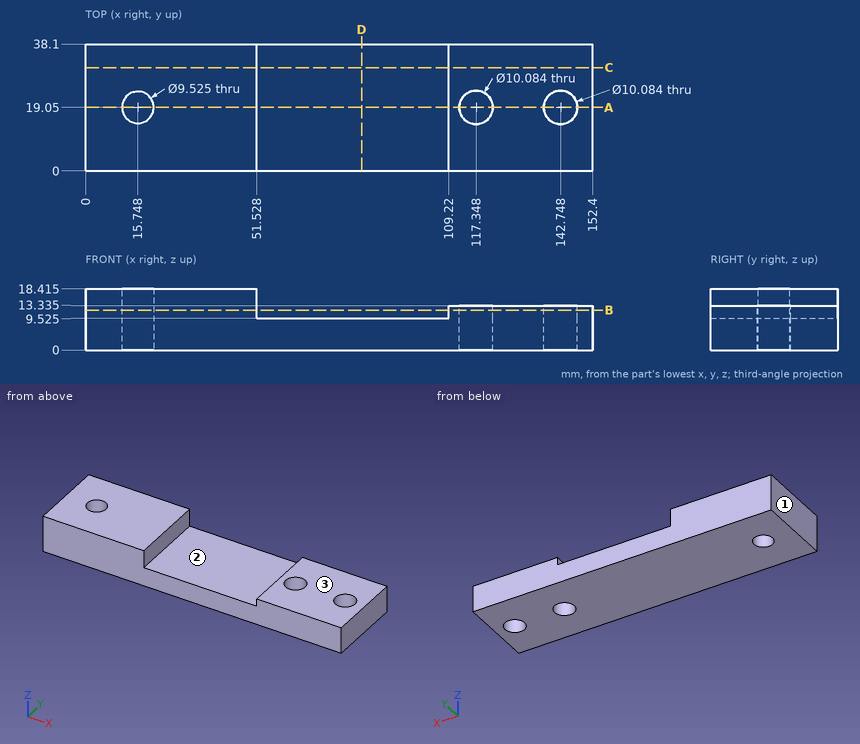
For this review, use the dimensioned drawing (mm, ordinates from the lowest corner) and the shaded views. A direction names the side the tool comes from. Round coordinates to 2 decimals unless told otherwise and drop trailing zeros. Write each loop counter-clockwise with the first axis right and the second up, starting at its lowest first coordinate (ties: lowest second). Pieces come first, ordered by that corner, then holes. Notation, with made-up numbers: (-1.75, -30.75) - (57.25, -30.75) arc R7 ccw to (57.25, -23.75) - close; hole circle Ø10 at (52, 23). An arc over 180 degrees is marked (long way). Use a Markdown table: item, result.
Q1. Machinability: for the marked faces 1, 2 and 3, which of the approach directions +Z, -Z, +X, -X, +Y, -Y give a long, thin tool a straight path to every point of the face, cutting with its end or side? Answer none if there is none.
Derived:
| item | result |
|---|---|
| face 1 | +Z, -Z, -X, +Y, -Y |
| face 2 | +Z, +Y, -Y |
| face 3 | +Z, +X, +Y, -Y |
Q2. We need section A-A (y = 19.05). Give the boundary of the cut face in (x, z) (1 decimal), plus the area to 3 significant figures.
Derived:
| item | result |
|---|---|
| outline | (0, 0) - (11, 0) - (11, 18.4) - (0, 18.4) - close; (20.5, 0) - (112.3, 0) - (112.3, 13.3) - (109.2, 13.3) - (109.2, 9.5) - (51.5, 9.5) - (51.5, 18.4) - (20.5, 18.4) - close; (122.4, 0) - (137.7, 0) - (137.7, 13.3) - (122.4, 13.3) - close; (147.8, 0) - (152.4, 0) - (152.4, 13.3) - (147.8, 13.3) - close |
| area | 1,630 mm2 |
Q3. We need section D-D (x = 83). Give the boundary of the cut face in (y, z) (1 decimal), plus the area to 3 significant figures.
Derived:
| item | result |
|---|---|
| outline | (0, 0) - (38.1, 0) - (38.1, 9.5) - (0, 9.5) - close |
| area | 363 mm2 |
Q4. Clearance check with flat-ended pins moving along their axes: pin 1 (16 mm diameter, centred on x = 142.748, y = 19.05, fed in from +Z) (3 decimals); pin 2 (9 mm diameter, centred on x = 117.348, y = 19.05, fed in from -Z). State where each tip first meets the part, or that it passes through.
Derived:
| item | result |
|---|---|
| pin 1 | stops at z = 13.335 |
| pin 2 | passes through |
Q5. Wall thickness on line 1 along X through (y, z) = (4, 10.5); line 2 along Z through (x, y) = (110.5, 27) (1 decimal); line 3 along Z through (x, y) = (52, 22.5) (1 decimal): over which ranges is each line inside the solid? List them lowest first.
Derived:
| item | result |
|---|---|
| line 1 | x = 0 to 51.53, 109.22 to 152.4 |
| line 2 | z = 0 to 13.3 |
| line 3 | z = 0 to 9.5 |
Q6. We need section C-C (y = 31). Give the boundary of the cut face in (x, z) (1 decimal).
Derived:
| item | result |
|---|---|
| outline | (0, 0) - (152.4, 0) - (152.4, 13.3) - (109.2, 13.3) - (109.2, 9.5) - (51.5, 9.5) - (51.5, 18.4) - (0, 18.4) - close |
Q7. We need section B-B (z = 12). State how many separate pieces and enclosed holes the cut face has, plus the area to 3 significant figures.
Derived:
| item | result |
|---|---|
| separate pieces | 2 |
| enclosed holes | 3 |
| area | 3,380 mm2 |
